Autodesk Inventor part; units mm, degrees
ref_plane "YZ Plane" through (0, 0, 0) normal (1, 0, 0) x (0, 1, 0)
ref_plane "XZ Plane" through (0, 0, 0) normal (0, 1, 0) x (-1, 0, 0)
ref_plane "XY Plane" through (0, 0, 0) normal (0, 0, 1) x (1, 0, 0)
sketch "スケッチ1" plane through (0, 0, 0) normal (0, 0, 1) x (1, 0, 0)
  line L0 (1.7321, -3) -> (-1.7321, -3)
  line L1 (-1.7321, -3) -> (-3.4641, 0)
  line L2 (-3.4641, 0) -> (-1.7321, 3)
  line L3 (-1.7321, 3) -> (1.7321, 3)
  line L4 (1.7321, 3) -> (3.4641, 0)
  line L5 (3.4641, 0) -> (1.7321, -3)
  point P0 (0, 0)
  point P1 (0, 0)
  dimension "d5" = 6
  dimension "d6" = 3
extrude "押し出し1" add sketch "スケッチ1" along normal blind 8
sketch "スケッチ2" plane through (0, 0, 8) normal (0, 0, 1) x (1, 0, 0)
  circle A0 centre (0, 0) radius 1.5
  dimension "d10" = 3
extrude "押し出し2" add sketch "スケッチ2" along normal blind 6
sketch "スケッチ3" plane through (0, 0, 0) normal (0, 0, -1) x (-1, 0, 0)
  circle A0 centre (0, 0) radius 1.5
  dimension "d13" = 3
hole "穴1" at (0, 0, 0) direction (0, 0, 1) diameter 3 depth 6 tip angle 118
thread "ねじ1"
thread "ねじ2"
fillet "フィレット1" radius 0.5 6 edges at (-3.4641, 0, 4) (-1.7321, -3, 4) (-1.7321, 3, 4) (1.7321, 3, 4) (3.4641, 0, 4) (1.7321, -3, 4)
Geometry check sheet. Reference: the model listing, model coordinates, mm. A direction names the side the tool comes from. Give positions to 0.01 mm unless a question says otherwise; leave off trailing zeros. Order: outer loops, then holes, each group sorted by start corner. A loop starts at its lowest first (then second) coordinate and runs counter-clockwise, first axis right, second up. Notation, with made-up numbers: (39, -9.5) - (43, -9.5) arc R12 ccw to (43, 6.5) - close; hole circle Ø4 at (62, 76.25). An arc over 180 degrees is marked (long way). Answer in a Markdown table with one row per item. Add a question column.
Q1. Cross-section at B-B, the plane z = 7.5. Enter the section's corners in (x, y), then the cut area to 3 significant figures.
Q2. Cross-section at A-A, the plane z = 4. Enter the section's corners in (x, y), then the cut area to 3 significant figures.
Q3. Tool access check on faces 4 (the flat face through (-2, 0, 8)), 5 (the flat face through (0, -3, 4)). Record the directions out of +Z, -Z, +X, -X, +Y, -Y that give a thin tool (end or side, any length) a straight path to the whole face; none if there is none.
Q4. Cross-section at C-C, the plane z = 11. Enter the section's corners in (x, y), then the cut area to 3 significant figures.
Q5. Mould release check, pull along X, two halves, no side actions. Record for faces 1 (the flat face through (0, 3, 4)), 2 (the cylindrical face through (-1.5, -0.07, 10.96)), 3 (the cylindrical face through (-0.07, -1.5, 3.04)): pulls with the +X half, pulls with the -X half, needs draft (parallel to the pull), parting line crosses it, or undercut.
Check values:
| question | item | result |
|---|---|---|
| 1 | outline | (-3.32, -0.25) - (-1.88, -2.75) arc R0.5 ccw to (-1.44, -3) - (1.44, -3) arc R0.5 ccw to (1.88, -2.75) - (3.32, -0.25) arc R0.5 ccw to (3.32, 0.25) - (1.88, 2.75) arc R0.5 ccw to (1.44, 3) - (-1.44, 3) arc R0.5 ccw to (-1.88, 2.75) - (-3.32, 0.25) arc R0.5 ccw to start |
| 1 | area | 31.1 mm^2 |
| 2 | outline | (-3.32, -0.25) - (-1.88, -2.75) arc R0.5 ccw to (-1.44, -3) - (1.44, -3) arc R0.5 ccw to (1.88, -2.75) - (3.32, -0.25) arc R0.5 ccw to (3.32, 0.25) - (1.88, 2.75) arc R0.5 ccw to (1.44, 3) - (-1.44, 3) arc R0.5 ccw to (-1.88, 2.75) - (-3.32, 0.25) arc R0.5 ccw to start; hole circle Ø3 at (0, 0) |
| 2 | area | 24.0 mm^2 |
| 3 | face 4 | +Z |
| 3 | face 5 | +Z, -Z, +X, -X, -Y |
| 4 | outline | circle Ø3 at (0, 0) |
| 4 | area | 7.07 mm^2 |
| 5 | face 1 | needs draft |
| 5 | face 2 | parting line crosses it |
| 5 | face 3 | undercut |
